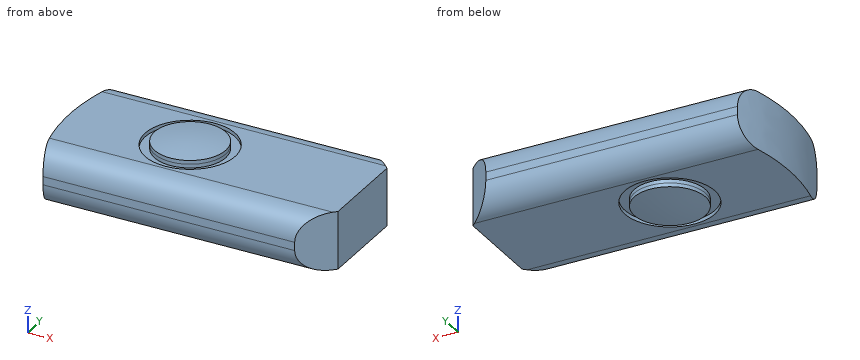
from build123d import *
from build123d.topology import SkipClean

# Parameters (mm, degrees)
BOSS_EXTRUDE1_DEPTH      = 7.7
FILLET1_R                = 3.3
CUT_EXTRUDE1_DEPTH       = 14.5
BOSS_EXTRUDE2_DEPTH      = 0.5
BOSS_EXTRUDE2_DEPTH_BACK = 8.2
SKETCH3_R                = 4.75
DOME1_FACE_RADIUS        = 4.75
DOME1_HEIGHT             = 0.5
DOME2_FACE_RADIUS        = 4.75
DOME2_HEIGHT             = 0.5
SKETCH4_R                = 6
SKETCH4_R_2              = 4.75
CUT_EXTRUDE2_DEPTH       = 0.5
CUT_EXTRUDE3_START       = -0.5
SKETCH5_R                = 6
SKETCH5_R_2              = 4.75
CUT_EXTRUDE3_DEPTH       = 0.5


with BuildPart() as part:
    # Sketch1 → Boss-Extrude1 (new body)
    with BuildSketch(Plane.XY):
        with BuildLine():
            Line((1.678605479, 0), (39, 0))
            Line((39, 0), (39, 19.5))
            Line((39, 19.5), (1.678605479, 19.5))
            add(Edge.make_bspline(
                [(1.678605479, 19.5), (-1.678605479, 9.75), (1.678605479, 0)],
                knots=[0, 0, 0, 1, 1, 1], degree=2))
        make_face()
    extrude(amount=BOSS_EXTRUDE1_DEPTH)

    # Fillet1
    fillet1_edges = [part.edges().sort_by_distance(p)[0] for p in [
        (20.339302739, 0, 7.7),
        (20.339302739, 0, 0),
        (20.339302739, 19.5, 0),
        (20.339302739, 19.5, 7.7),
    ]]
    fillet(fillet1_edges, radius=FILLET1_R)

    # Sketch2 → Cut-Extrude1 (cut)
    with BuildSketch(Plane.XY):
        Polygon((35.25816866, 19.5), (39, 15.75816866), (39, 3.74183134), (35.25816866, 0), (41.546520984, 0), (41.546520984, 19.5), align=None)
    extrude(amount=CUT_EXTRUDE1_DEPTH, mode=Mode.SUBTRACT)

    # Sketch3 → Boss-Extrude2 (add, two sides: drawn at the far end of the back side and taken through both)
    with BuildSketch(Plane.XY.offset(7.7).offset(-BOSS_EXTRUDE2_DEPTH_BACK)):
        with Locations((16, 9.75)):
            Circle(SKETCH3_R)
    extrude(amount=BOSS_EXTRUDE2_DEPTH + BOSS_EXTRUDE2_DEPTH_BACK)

    # Dome1: a dome of height H over a round flat face of radius A is a cap of a sphere of radius (A * A + H * H) / (2 * H)
    dome1_r = (DOME1_FACE_RADIUS * DOME1_FACE_RADIUS + DOME1_HEIGHT * DOME1_HEIGHT) / (2 * DOME1_HEIGHT)
    dome1_base = Plane((16, 9.75, 8.2), z_dir=(0, 0, 1))
    with Locations(dome1_base.offset(DOME1_HEIGHT - dome1_r)):
        dome1_ball = Sphere(dome1_r, mode=Mode.PRIVATE)
    add(split(dome1_ball, bisect_by=dome1_base, keep=Keep.TOP, mode=Mode.PRIVATE))

    # Dome2: a dome of height H over a round flat face of radius A is a cap of a sphere of radius (A * A + H * H) / (2 * H)
    dome2_r = (DOME2_FACE_RADIUS * DOME2_FACE_RADIUS + DOME2_HEIGHT * DOME2_HEIGHT) / (2 * DOME2_HEIGHT)
    dome2_base = Plane((16, 9.75, -0.5), z_dir=(0, 0, -1))
    with Locations(dome2_base.offset(DOME2_HEIGHT - dome2_r)):
        dome2_ball = Sphere(dome2_r, mode=Mode.PRIVATE)
    add(split(dome2_ball, bisect_by=dome2_base, keep=Keep.TOP, mode=Mode.PRIVATE))

    # Sketch4 → Cut-Extrude2 (cut)
    with BuildSketch(Plane(origin=(0, 0, 0), x_dir=(-1, 0, 0), z_dir=(0, 0, -1))):
        with Locations((-16, 9.75)):
            Circle(SKETCH4_R)
        with Locations(Location((-16, 9.75, 0), (0, 0, 180))):
            Circle(SKETCH4_R_2, mode=Mode.SUBTRACT)
    extrude(amount=-CUT_EXTRUDE2_DEPTH, mode=Mode.SUBTRACT)

    # Sketch5 → Cut-Extrude3 (cut)
    with SkipClean():  # the faces are left unmerged after this step: merging them gives an invalid solid
        with BuildSketch(Plane.XY.offset(7.7).offset(CUT_EXTRUDE3_START)):
            with Locations(Location((16, 9.75, 0), (0, 0, 180))):
                Circle(SKETCH5_R)
            with Locations((16, 9.75)):
                Circle(SKETCH5_R_2, mode=Mode.SUBTRACT)
        extrude(amount=CUT_EXTRUDE3_DEPTH, mode=Mode.SUBTRACT)


solid = part.part
For this review, take the finished solid that the model builds, in its own axes (mm). Round coordinates to 2 decimals unless told otherwise and drop trailing zeros. Order: outer loops, then holes, each group sorted by start corner. A loop starts at its lowest first (then second) coordinate and runs counter-clockwise, first axis right, second up. Notation, with made-up numbers: M -5.75,-8.75 L 21.25,-8.75 A30 ccw 21.25,28.25 Z; hole C -8,12.25 d8. An arc over 180 degrees is marked long. Use a Markdown table: item, result. Add a question column.
Item 1: Insertion check: pin 1 (3.5 mm diameter, centred on x = 17.5, y = 12, fed in from -Z); pin 2 (8 mm diameter, centred on x = 13.5, y = 4, fed in from +Z); pin 3 (5 mm diameter, centred on x = 20, y = 14, fed in from -Z). Each pin has a flat end and moves straight along its axis. Give the tip position at first contact, or say it passes through.
Item 2: To check wall thickness, follow line 1 along Y through (x, z) = (16, 7.3); line 2 along Z through (x, y) = (13, 3.5); line 3 along Y through (x, z) = (16, 4.5). State the ranges of each line that lie inside material, in increasing order.
Item 3: Add section A-A, the plane x = 3. Give the boundary of the cut face in (y, z), then the cut area to 3 significant figures.
Geometry results:
| question | item | result |
|---|---|---|
| 1 | pin 1 | stops at z = -0.98 |
| 1 | pin 2 | stops at z = 8.59 |
| 1 | pin 3 | stops at z = -0.75 |
| 2 | line 1 | y = 1.73 to 3.75, 5 to 14.5, 15.75 to 17.77 |
| 2 | line 2 | z = 0 to 7.7 |
| 2 | line 3 | y = 0 to 19.5 |
| 3 | outline | M 0,3.3 A3.3 ccw 3.3,0 L 16.2,0 A3.3 ccw 19.5,3.3 L 19.5,4.4 A3.3 ccw 16.2,7.7 L 3.3,7.7 A3.3 ccw 0,4.4 Z |
| 3 | area | 141 mm² |
